```python
from build123d import *

# Parameters (mm, degrees)
SWEEP1_PROFILE_R   = 3
SKETCH3_R          = 1.6
CUT_EXTRUDE1_DEPTH = 7


with BuildPart() as part:
    # Sweep1: sweep along a path in Sketch2
    with BuildLine(Plane.XY) as sweep1_path:
        Line((0, 0), (10, 0))
        Line((10, 0), (18.119816674, 5.836829378))
    # Sweep1 profile (on start of the path) → Sweep1 (sweep)
    with BuildSketch(Plane(origin=(0, 0, 0), x_dir=(0, 0, 1), z_dir=(1, 0, 0))):
        Circle(SWEEP1_PROFILE_R)
    sweep(path=sweep1_path.line, transition=Transition.RIGHT)

    # Sketch3 → Cut-Extrude1 (cut)
    with BuildSketch(Plane(origin=(0, 0, 0), x_dir=(0, 0, -1), z_dir=(1, 0, 0))):
        Circle(SKETCH3_R)
    cut_extrude1 = extrude(amount=CUT_EXTRUDE1_DEPTH, mode=Mode.SUBTRACT)

    # Mirror1: Cut-Extrude1 across plane
    add(cut_extrude1.mirror(Plane(origin=(9.059908337, 2.918414689, 0), x_dir=(0, 0, 1), z_dir=(0.951835508, 0.306609143, 0))), mode=Mode.SUBTRACT)


solid = part.part
```
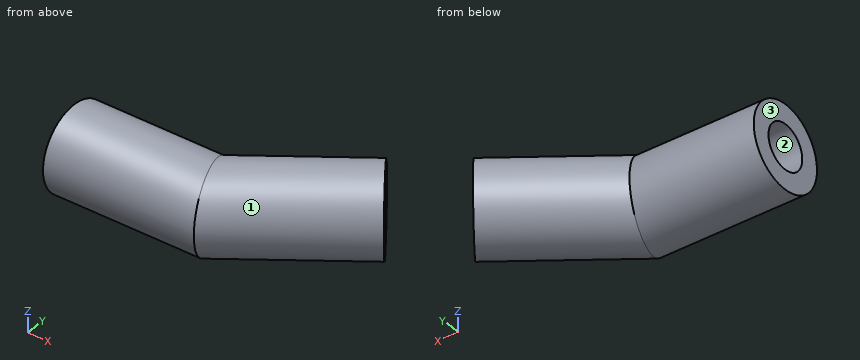
For this review, take the finished solid that the model builds, in its own axes (mm). Face numbers are marked on the shaded views. Give positions to 0.01 mm unless a question says otherwise; leave off trailing zeros. Write each loop counter-clockwise with the first axis right and the second up, starting at its lowest first coordinate (ties: lowest second). Pieces come first, ordered by that corner, then holes.
Item 1: Insertion check: P1, Ø6, axis at x = 8.5, y = 4, coming from the +Z side; P2, Ø5, axis at x = 14.5, y = 7, coming from the -Z side. Each pin has a flat end and moves straight along its axis. Give the tip position at first contact, or say it passes through.
Item 2: Take a section at C-C (z = -1.1). Give the boundary of the cut face in (x, y).
Item 3: Wall thickness on probe 1 along Y at (x, z) = (3.75, 0); probe 2 along X at (y, z) = (1.5, -1.1); probe 3 along Z at (x, y) = (16.75, 3): over which ranges is each line inside the solid? List them lowest first.
Item 4: Take a section at A-A (z = 0.9). Give the boundary of the cut face in (x, y).
Item 5: The part is to be moulded in two halves that separate along Y. For the marked faces 1, 2 and 3, say which applies: +Y half, -Y half, draft (parallel to the pull), parting line (faces both ways), or undercut.
Item 6: Take a section at B-B (x = 7.75). Give the boundary of the cut face in (y, z), and give its area (3 significant figures).
Established:
1. P1: stops at z = 2.83
1. P2: stops at z = -2.95
2. outline: (0, -2.79) - (10.9, -2.79) - (19.75, 3.57) - (18.8, 4.89) - (13.11, 0.81) - (11.76, 2.69) - (17.44, 6.78) - (16.49, 8.1) - (9.1, 2.79) - (0, 2.79) - (0, 1.16) - (7, 1.16) - (7, -1.16) - (0, -1.16) - close
3. probe 1: y = -3 to -1.6, 1.6 to 3
3. probe 2: x = 0 to 12.62, 14.08 to 16.87
3. probe 3: z = -2.6 to -0.55, 0.55 to 2.6
4. outline: (0, -2.86) - (10.92, -2.86) - (19.79, 3.51) - (18.89, 4.76) - (13.21, 0.68) - (11.66, 2.83) - (17.35, 6.91) - (16.45, 8.16) - (9.08, 2.86) - (0, 2.86) - (0, 1.32) - (7, 1.32) - (7, -1.32) - (0, -1.32) - close
5. face 1: parting line
5. face 2: undercut
5. face 3: draft
6. outline: circle Ø6 at (0, 0)
6. area: 28.3 mm2
